from build123d import *

# Parameters (mm, degrees)
SKETCH1_R           = 1.55
SKETCH1_R_2         = 2.97333552
SKETCH1_R_3         = 2.85410663
BOSS_EXTRUDE1_DEPTH = 3.175
CUT_EXTRUDE1_DEPTH  = 3.175


with BuildPart() as part:
    # Sketch1 → Boss-Extrude1 (new body)
    with BuildSketch(Plane(origin=(0, 0, 0), x_dir=(1, 0, 0), z_dir=(0, 1, 0))):
        with BuildLine():
            Line((-15.352336135, 71.529843551), (-126.166636901, 37.820307959))
            Line((-126.166636901, 37.820307959), (-126.166636901, 31.407196795))
            Line((-126.166636901, 31.407196795), (-147.248636901, 31.407196795))
            Line((-147.248636901, 31.407196795), (-150.296636901, 30.48))
            Line((-150.296636901, 30.48), (-150.296636901, 17.78))
            Line((-150.296636901, 17.78), (-74.096636901, 17.78))
            ThreePointArc((-74.096636901, 17.78), (-76.2, 0), (-74.096636901, -17.78))
            Line((-74.096636901, -17.78), (-150.296636901, -17.78))
            Line((-150.296636901, -17.78), (-150.296636901, -30.48))
            Line((-150.296636901, -30.48), (-147.248636901, -31.407196795))
            Line((-147.248636901, -31.407196795), (-126.166636901, -31.407196795))
            Line((-126.166636901, -31.407196795), (-126.166636901, -37.820307959))
            Line((-126.166636901, -37.820307959), (-15.352336135, -71.529843551))
            Line((-15.352336135, -71.529843551), (-15.352336135, -58.127428782))
            Line((-15.352336135, -58.127428782), (15.24, -58.127428782))
            Line((15.24, -58.127428782), (15.24, -74.66044736))
            ThreePointArc((15.24, -74.66044736), (76.2, 0), (15.24, 74.66044736))
            Line((15.24, 74.66044736), (15.24, 58.127428782))
            Line((15.24, 58.127428782), (-15.352336135, 58.127428782))
            Line((-15.352336135, 58.127428782), (-15.352336135, 71.529843551))
        make_face()
        with Locations((-56.1402016, 0)):
            Circle(SKETCH1_R, mode=Mode.SUBTRACT)
        with Locations((-19.5642016, -23.368)):
            Circle(SKETCH1_R, mode=Mode.SUBTRACT)
        with Locations((64.77, -19.558)):
            Circle(SKETCH1_R_2, mode=Mode.SUBTRACT)
        with Locations((16.51, -13.97)):
            Circle(SKETCH1_R, mode=Mode.SUBTRACT)
        with Locations((44.45, -13.97)):
            Circle(SKETCH1_R, mode=Mode.SUBTRACT)
        with Locations((-147.248636901, 27.94)):
            Circle(SKETCH1_R, mode=Mode.SUBTRACT)
        with Locations((-126.166636901, 27.94)):
            Circle(SKETCH1_R, mode=Mode.SUBTRACT)
        with Locations((-56.1402016, 34.29)):
            Circle(SKETCH1_R, mode=Mode.SUBTRACT)
        with Locations((16.51, 13.97)):
            Circle(SKETCH1_R, mode=Mode.SUBTRACT)
        with Locations((44.45, 13.97)):
            Circle(SKETCH1_R, mode=Mode.SUBTRACT)
        with Locations((64.77, 19.558)):
            Circle(SKETCH1_R_3, mode=Mode.SUBTRACT)
        with Locations((-19.5642016, 23.368)):
            Circle(SKETCH1_R, mode=Mode.SUBTRACT)
        with Locations((-56.1402016, -34.29)):
            Circle(SKETCH1_R, mode=Mode.SUBTRACT)
        with Locations((-126.166636901, -27.94)):
            Circle(SKETCH1_R, mode=Mode.SUBTRACT)
        with Locations((-147.248636901, -27.94)):
            Circle(SKETCH1_R, mode=Mode.SUBTRACT)
    extrude(amount=BOSS_EXTRUDE1_DEPTH)

    # Sketch2 → Cut-Extrude1 (cut)
    with BuildSketch(Plane(origin=(0, 3.175, 0), x_dir=(1, 0, 0), z_dir=(0, 1, 0))):
        Polygon((-126.166636901, 31.407196795), (-68.501735058, 45.311715833), (-70.759486518, 54.675075755), (-126.166636901, 37.820307959), align=None)
        Polygon((-68.501735058, -45.311715833), (-126.166636901, -31.407196795), (-126.166636901, -37.820307959), (-70.759486518, -54.675075755), align=None)
    extrude(amount=-CUT_EXTRUDE1_DEPTH, mode=Mode.SUBTRACT)


solid = part.part
Work out the finished part from the listing and answer in its coordinate system (mm). Give positions to 0.01 mm unless a question says otherwise; leave off trailing zeros. Loops run counter-clockwise (first coordinate to the right, second up) from the corner with the lowest first, then second, coordinate; pieces in that order, holes last. Notation, with made-up numbers: (80, 7.25) - (130, 7.25) arc R17 ccw to (130, 14.25) - close; hole circle Ø11 at (7.25, 54). An arc over 180 degrees is marked (long way). Answer in a Markdown table with one row per item. Add a question column.
Q1. Consider line 1 along Z through (x, y) = (44.45, 1.6); line 2 along X through (y, z) = (0.35, 13.5); line 3 along X through (y, z) = (1.2, -28.5). Determine where each line is inside the solid, lowest interval first.
Q2. Determine the mould class of faces 1 (the flat face through (-13, 3.175, -1)), 2 (the cylindrical face through (62.579, 1.565, 17.548)), 3 (the flat face through (-42.67, 1.57, -63.22)) for opening direction Z: released by +Z, released by -Z, zero draft, split by the parting line, or undercut.
Q3. The part is cut by section B-B (x = 64.77). Determine the outline of the cut face in (y, z) (3 decimals), and give its area (3 significant figures).
Q4. The part is cut by section D-D (y = 2.15). State how many separate pieces and enclosed holes the cut face has, and give its area (3 significant figures).
Q5. Each of these flat-tipped pins is pushed along its axis until it touches: P1, Ø1, axis at x = -121.5, y = 2.5, coming from the -Z side; P2, Ø3, axis at x = -56.14, z = 0, coming from the +Y side; P3, Ø1.5, axis at x = -68.5, y = 1, coming from the -Z side; P4, Ø1, axis at x = -80.5, y = 2, coming from the +Z side. Where does it stop, or does it pass through?
Q6. The part is cut by section C-C (z = -61.5). Determine the outline of the cut face in (x, y) (3 decimals).
Q7. The part is cut by section A-A (x = -111). Determine the outline of the cut face in (y, z) (3 decimals).
Solution:
| question | item | result |
|---|---|---|
| 1 | line 1 | z = -61.89 to -15.52, -12.42 to 12.42, 15.52 to 61.89 |
| 1 | line 2 | x = -74.99 to 15.03, 17.99 to 42.97, 45.93 to 74.99 |
| 1 | line 3 | x = -150.3 to -148.69, -145.8 to -127.61, -124.72 to 70.67 |
| 2 | face 1 | zero draft |
| 2 | face 2 | undercut |
| 2 | face 3 | released by -Z |
| 3 | outline | (0, -40.141) - (3.175, -40.141) - (3.175, -22.412) - (0, -22.412) - close; (0, -16.704) - (3.175, -16.704) - (3.175, 16.585) - (0, 16.585) - close; (0, 22.531) - (3.175, 22.531) - (3.175, 40.141) - (0, 40.141) - close |
| 3 | area | 218 mm² |
| 4 | separate pieces | 1 |
| 4 | enclosed holes | 15 |
| 4 | area | 20,300 mm² |
| 5 | P1 | stops at z = -32.65 |
| 5 | P2 | passes through |
| 5 | P3 | stops at z = -55.59 |
| 5 | P4 | stops at z = 42.54 |
| 6 | outline | (-48.324, 0) - (-15.352, 0) - (-15.352, 3.175) - (-48.324, 3.175) - close; (15.24, 0) - (44.991, 0) - (44.991, 3.175) - (15.24, 3.175) - close |
| 7 | outline | (0, -35.064) - (3.175, -35.064) - (3.175, -17.78) - (0, -17.78) - close; (0, 17.78) - (3.175, 17.78) - (3.175, 35.064) - (0, 35.064) - close |
